Check sheet for the modelled part. Datum: model origin and axes. Units: mm. A direction names the side the tool comes from. Coordinates: 2 decimals unless noted, no trailing zeros. Loops run counter-clockwise (first coordinate to the right, second up) from the corner with the lowest first, then second, coordinate; pieces in that order, holes last.
```python
from build123d import *

# Parameters (mm, degrees)
SKETCH1_R           = 1.5
SKETCH1_R_2         = 10
SKETCH1_R_3         = 1.494637137
SKETCH1_W           = 25
SKETCH1_H           = 20
SKETCH1_W_2         = 12
BOSS_EXTRUDE2_DEPTH = 5
SKETCH2_R           = 1.5
CUT_EXTRUDE1_DEPTH  = 100
SKETCH3_R           = 1.5
CUT_EXTRUDE2_DEPTH  = 1220
SKETCH5_R           = 1.5
CUT_EXTRUDE4_DEPTH  = 10


with BuildPart() as part:
    # Sketch1 → Boss-Extrude2 (new body)
    with BuildSketch(Plane(origin=(0, 0, 0), x_dir=(1, 0, 0), z_dir=(0, 1, 0))):
        Polygon((0, 0), (130, 0), (130, 185), (110, 185), (110, 150), (35, 150), (35, 185), (0, 185), align=None)
        with Locations(Location((126, 4, 0), (0, 0, 270))):
            Circle(SKETCH1_R, mode=Mode.SUBTRACT)
        with Locations(Location((4, 4, 0), (0, 0, 90))):
            Circle(SKETCH1_R, mode=Mode.SUBTRACT)
        with Locations(Location((4, 181, 0), (0, 0, 270))):
            Circle(SKETCH1_R, mode=Mode.SUBTRACT)
        with Locations(Location((126, 181, 0), (0, 0, 90))):
            Circle(SKETCH1_R, mode=Mode.SUBTRACT)
        with Locations(Location((13, 80, 0), (0, 0, 270))):
            Circle(SKETCH1_R_2, mode=Mode.SUBTRACT)
        with Locations(Location((118, 80, 0), (0, 0, 270))):
            Circle(SKETCH1_R_2, mode=Mode.SUBTRACT)
        with Locations(Location((79.5, 107.5, 0), (0, 0, 270))):
            Circle(SKETCH1_R, mode=Mode.SUBTRACT)
        with Locations(Location((50, 107.5, 0), (0, 0, 270))):
            Circle(SKETCH1_R, mode=Mode.SUBTRACT)
        with Locations(Location((20.081102583, 128.469773312, 0), (0, 0, 270))):
            Circle(SKETCH1_R_3, mode=Mode.SUBTRACT)
        with Locations(Location((116.797060631, 180.536614994, 0), (0, 0, 270))):
            Circle(SKETCH1_R, mode=Mode.SUBTRACT)
        with Locations(Location((20.081102583, 182.469773312, 0), (0, 0, 270))):
            Circle(SKETCH1_R, mode=Mode.SUBTRACT)
        with Locations(Location((116.797060631, 160.536614994, 0), (0, 0, 270))):
            Circle(SKETCH1_R, mode=Mode.SUBTRACT)
        with Locations((64.5, 100)):
            Rectangle(SKETCH1_W, SKETCH1_H, mode=Mode.SUBTRACT)
        with Locations((11, 110)):
            Rectangle(SKETCH1_W_2, SKETCH1_H, mode=Mode.SUBTRACT)
        with Locations((121, 110)):
            Rectangle(SKETCH1_W_2, SKETCH1_H, mode=Mode.SUBTRACT)
        with Locations((121, 140)):
            Rectangle(SKETCH1_W_2, SKETCH1_H, mode=Mode.SUBTRACT)
    extrude(amount=BOSS_EXTRUDE2_DEPTH)

    # Sketch2 → Cut-Extrude1 (cut)
    with BuildSketch(Plane(origin=(0, 5, 0), x_dir=(1, 0, 0), z_dir=(0, 1, 0))):
        with Locations(Location((12.444428106, 65.171668427, 0), (0, 0, 270))):
            Circle(SKETCH2_R)
        with Locations(Location((91.184428106, 65.171668427, 0), (0, 0, 90))):
            Circle(SKETCH2_R)
        with Locations(Location((91.184428106, 9.291668427, 0), (0, 0, 270))):
            Circle(SKETCH2_R)
        with Locations(Location((12.444428106, 9.291668427, 0), (0, 0, 90))):
            Circle(SKETCH2_R)
    extrude(amount=-CUT_EXTRUDE1_DEPTH, mode=Mode.SUBTRACT)

    # Sketch3 → Cut-Extrude2 (cut)
    with BuildSketch(Plane(origin=(0, 5, 0), x_dir=(1, 0, 0), z_dir=(0, 1, 0))):
        with Locations(Location((108.6, 61.26, 0), (0, 0, 270))):
            Circle(SKETCH3_R)
        with Locations(Location((107.33, 13, 0), (0, 0, 270))):
            Circle(SKETCH3_R)
        with Locations(Location((32.4, 13, 0), (0, 0, 270))):
            Circle(SKETCH3_R)
        with Locations(Location((26.1, 61.26, 0), (0, 0, 270))):
            Circle(SKETCH3_R)
        with Locations(Location((56.53, 56.18, 0), (0, 0, 270))):
            Circle(SKETCH3_R)
        with Locations(Location((56.5, 28.1, 0), (0, 0, 270))):
            Circle(SKETCH3_R)
    extrude(amount=-CUT_EXTRUDE2_DEPTH, mode=Mode.SUBTRACT)

    # Sketch5 → Cut-Extrude4 (cut)
    with BuildSketch(Plane(origin=(0, 5, 0), x_dir=(1, 0, 0), z_dir=(0, 1, 0))):
        with Locations(Location((37.2, 120, 0), (0, 0, 270))):
            Circle(SKETCH5_R)
        with Locations(Location((106, 120, 0), (0, 0, 90))):
            Circle(SKETCH5_R)
        with Locations(Location((106, 68, 0), (0, 0, 270))):
            Circle(SKETCH5_R)
        with Locations(Location((37.2, 68, 0), (0, 0, 90))):
            Circle(SKETCH5_R)
    extrude(amount=-CUT_EXTRUDE4_DEPTH, mode=Mode.SUBTRACT)


solid = part.part
```
1) Section check B-B on x = 43. Enter the section's corners in (y, z), plus the area to 3 significant figures.
Answer sheet:
outline: (0, -150) - (5, -150) - (5, 0) - (0, 0) - close
area: 750 mm2
2) Section check A-A on z = -80. Enter the section's corners in (x, y).
Answer sheet:
outline: (0, 0) - (3, 0) - (3, 5) - (0, 5) - close; (23, 0) - (108, 0) - (108, 5) - (23, 5) - close; (128, 0) - (130, 0) - (130, 5) - (128, 5) - close
3) Mould release check, pull along X, two halves, no side actions. Record for faces 1 (the flat face through (11, 2, -100)), 2 (the flat face through (120, 2, -185)), 3 (the flat face through (73, 2, -150)), 4 (the flat face through (130, 2, -91)): +X half, -X half, draft (parallel to the pull), parting line (faces both ways), or undercut.
Answer sheet:
face 1: undercut
face 2: draft
face 3: undercut
face 4: +X half
4) Set-up check for faces 5 (the flat face through (110, 2, -168)), 6 (the flat face through (64, 5, -73)), 7 (the flat face through (127, 2, -140)): record each of +Z, -Z, +X, -X, +Y, -Y from which the full face is reachable in a straight line by a thin tool's end or side.
Answer sheet:
face 5: -Z, +Y, -Y
face 6: +Z, -Z, +X, -X, +Y
face 7: +Y, -Y
5) Depth check by flat-ended pin: pin 1 (4 mm diameter, centred on x = 20.08, z = -182.47, fed in from -Y). Enter the tip coordinate at first touch or a pass-through.
Answer sheet:
pin 1: stops at y = 0
6) Section check C-C on y = 3.05. Give the number of separate pieces and of enclosed holes in the cut face, plus the area to 3 significant figures.
Answer sheet:
separate pieces: 1
enclosed holes: 30
area: 19,400 mm2
7) Scan lines: line 1 (X direction, y = 4.5, z = -9); line 2 (X direction, y = 3.85, z = -13); line 3 (X direction, y = 1, z = -102). Record each from-to range of solid material in increasing order.
Answer sheet:
line 1: x = 0 to 10.97, 13.92 to 89.71, 92.66 to 130
line 2: x = 0 to 30.9, 33.9 to 105.83, 108.83 to 130
line 3: x = 0 to 5, 17 to 52, 77 to 115, 127 to 130
